from build123d import *

# Parameters (mm, degrees)
SKETCH1_R                                            = 20
SKETCH1_R_2                                          = 12.5
SKETCH1_W                                            = 15
SKETCH1_H                                            = 150
BOSS_EXTRUDE1_DEPTH                                  = 6
SKETCH2_R                                            = 6.5
CUT_EXTRUDE1_DEPTH                                   = 6
FILLET1_R                                            = 10
CBORE_FOR_M3_HEX_SOCKET_HEAD_CAP_SCREW2_D            = 3.4
CBORE_FOR_M3_HEX_SOCKET_HEAD_CAP_SCREW2_CBORE_D      = 6.5
CBORE_FOR_M3_HEX_SOCKET_HEAD_CAP_SCREW2_CBORE_DEPTH  = 3.4
CIRPATTERN1_COUNT                                    = 6
CSK_FOR_M3_HEX_SOCKET_COUNTERSUNK_CAP_SC_D           = 3.4
CSK_FOR_M3_HEX_SOCKET_COUNTERSUNK_CAP_SC_CSINK_D     = 6.72
CSK_FOR_M3_HEX_SOCKET_COUNTERSUNK_CAP_SC_CSINK_ANGLE = 90
CHAMFER1_SIZE                                        = 1


with BuildPart() as part:
    # Sketch1 → Boss-Extrude1 (new body)
    with BuildSketch(Plane.XY):
        with Locations((0, 75)):
            Circle(SKETCH1_R)
        with Locations((0, -75)):
            Circle(SKETCH1_R_2)
        Rectangle(SKETCH1_W, SKETCH1_H)
    extrude(amount=BOSS_EXTRUDE1_DEPTH)

    # Sketch2 → Cut-Extrude1 (cut)
    with BuildSketch(Plane.XY.offset(6)):
        with Locations((0, 68)):
            Circle(SKETCH2_R)
    extrude(amount=-CUT_EXTRUDE1_DEPTH, mode=Mode.SUBTRACT)

    # Fillet1
    fillet1_edges = [part.edges().sort_by_distance(p)[0] for p in [
        (7.5, 56.459503782, 3),
        (7.5, -65, 3),
        (-7.5, -65, 3),
        (-7.5, 56.459503782, 3),
    ]]
    fillet(fillet1_edges, radius=FILLET1_R)

    # CBORE for M3 Hex Socket Head Cap Screw2 (through all)
    with Locations(Plane(origin=(15.5, 75, 6), x_dir=(1, 0, 0), z_dir=(0, 0, 1))):
        with Locations((0, 0)):
            cbore_for_m3_hex_socket_head_cap_screw2 = CounterBoreHole(CBORE_FOR_M3_HEX_SOCKET_HEAD_CAP_SCREW2_D / 2, CBORE_FOR_M3_HEX_SOCKET_HEAD_CAP_SCREW2_CBORE_D / 2, CBORE_FOR_M3_HEX_SOCKET_HEAD_CAP_SCREW2_CBORE_DEPTH)

    # CirPattern1: CBORE for M3 Hex Socket Head Cap Screw2 ×6 about axis
    cirpattern1_axis = Axis((0, 75, 0), (0, 0, 1))
    for i in range(1, CIRPATTERN1_COUNT):
        add(cbore_for_m3_hex_socket_head_cap_screw2.rotate(cirpattern1_axis, i * 360 / CIRPATTERN1_COUNT), mode=Mode.SUBTRACT)

    # CSK for M3 Hex Socket Countersunk Cap Screw1 (through all)
    with Locations(Plane(origin=(0, -67, 6), x_dir=(1, 0, 0), z_dir=(0, 0, 1))):
        with Locations((0, 0), (8, -8), (0, -16), (-8, -8)):
            CounterSinkHole(CSK_FOR_M3_HEX_SOCKET_COUNTERSUNK_CAP_SC_D / 2, CSK_FOR_M3_HEX_SOCKET_COUNTERSUNK_CAP_SC_CSINK_D / 2, counter_sink_angle=CSK_FOR_M3_HEX_SOCKET_COUNTERSUNK_CAP_SC_CSINK_ANGLE)

    # Chamfer1
    chamfer1_edges = [part.edges().sort_by_distance(p)[0] for p in [
        (7.5, -5.112425119, 0),
        (7.5, -5.112425119, 6),
        (0, -87.5, 0),
        (0, -87.5, 6),
        (-7.5, -5.112425119, 0),
        (-7.5, -5.112425119, 6),
        (0, 95, 0),
        (0, 95, 6),
        (8.071909584, -64.19119771, 0),
        (8.071909584, -64.19119771, 6),
        (-8.071909584, -64.19119771, 0),
        (-8.071909584, -64.19119771, 6),
        (-8.60243479, 55.197368784, 0),
        (-8.60243479, 55.197368784, 6),
        (8.60243479, 55.197368784, 0),
        (8.60243479, 55.197368784, 6),
    ]]
    chamfer(chamfer1_edges, length=CHAMFER1_SIZE)


solid = part.part
Verification items for the finished model (mm, model axes). A direction names the side the tool comes from. Coordinates: 2 decimals unless noted, no trailing zeros. Order: outer loops, then holes, each group sorted by start corner. A loop starts at its lowest first (then second) coordinate and runs counter-clockwise, first axis right, second up.
1. Scan lines: line 1 (X direction, y = -75, z = 2.95); line 2 (X direction, y = 73, z = 3.45); line 3 (Y direction, x = -0.5, z = 5.6). Record each from-to range of solid material in increasing order.
Results found:
line 1: x = -12.5 to -9.7, -6.3 to 6.3, 9.7 to 12.5
line 2: x = -19.9 to -18.06, -12.94 to -4.15, 4.15 to 12.94, 18.06 to 19.9
line 3: y = -86.89 to -85.92, -80.08 to -69.92, -64.08 to 61.52, 74.48 to 94.39
2. Set-up check for faces 3 (the face through (8.173, 58.354, 4.324)), 4 (the face through (-8.66, 89.86, 1.28)), 5 (the face through (8.633, 55.256, 3.028)): record each of +Z, -Z, +X, -X, +Y, -Y from which the full face is reachable in a straight line by a thin tool's end or side.
Results found:
face 3: +Z
face 4: +Z, -Z
face 5: +Z, -Z, +X
3. Sectioned sample at B-B, the plane y = 1.5. Record the cut outline in (x, z), and give its area (3 significant figures).
Results found:
outline: (-7.5, 1) - (-6.5, 0) - (6.5, 0) - (7.5, 1) - (7.5, 5) - (6.5, 6) - (-6.5, 6) - (-7.5, 5) - close
area: 88.0 mm2
4. Release check for a two-part mould opening along Y. For faces 1 (the face through (0, 5, 6)), 2 (the face through (7.381, 90.083, 1.282)) record: +Y half, -Y half, draft (parallel to the pull), parting line (faces both ways), or undercut.
Results found:
face 1: draft
face 2: undercut
5. Sectioned sample at A-A, the plane x = 0. Record the cut outline in (y, z).
Results found:
outline: (-87.5, 1) - (-86.5, 0) - (-84.7, 0) - (-84.7, 4.34) - (-86.36, 6) - (-86.5, 6) - (-87.5, 5) - close; (-81.3, 0) - (-68.7, 0) - (-68.7, 4.34) - (-70.36, 6) - (-79.64, 6) - (-81.3, 4.34) - close; (-65.3, 0) - (61.5, 0) - (61.5, 6) - (-63.64, 6) - (-65.3, 4.34) - close; (74.5, 0) - (94, 0) - (95, 1) - (95, 5) - (94, 6) - (74.5, 6) - close
6. Go/stop test with flat-tipped pins: pin 1 Ø1 at (x, z) = (-10, 1) entering from -Y; pin 2 Ø1 at (x, z) = (3.5, 2) entering from -Y; pin 3 Ø4 at (x, y) = (7.75, 61.58) entering from -Z; pin 4 Ø5 at (x, y) = (8, 89) entering from +Z. Record where each tip stops, or that it passes through.
Results found:
pin 1: stops at y = -83.12
pin 2: stops at y = -87.13
pin 3: stops at z = 0
pin 4: stops at z = 2.6
